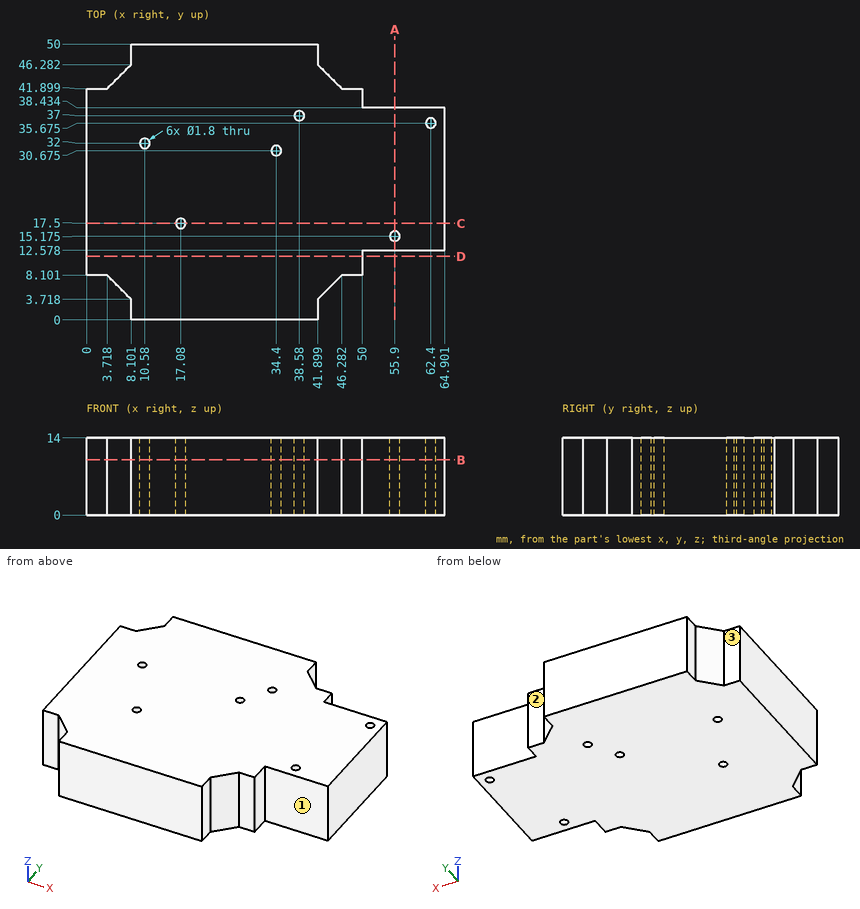
Job drawing, mm, ordinate dimensions from the low corner. One solid piece. A direction names the side the tool comes from. Give positions to 0.01 mm unless a question says otherwise; leave off trailing zeros. Loops run counter-clockwise (first coordinate to the right, second up) from the corner with the lowest first, then second, coordinate; pieces in that order, holes last. Notation, with made-up numbers: M 61.5,64 L 119.5,64 A18 ccw 119.5,96 Z; hole C 19.25,45.25 d1. An arc over 180 degrees is marked long. Put each result on its own line as item: value. Start each with the question number.
1) Saw through at D-D (y = 11.5). List the corners of the cut face in (x, z).
2) Saw through at A-A (x = 55.9). List the corners of the cut face in (y, z) (1 decimal).
3) Saw through at C-C (y = 17.5). List the corners of the cut face in (x, z).
4) 3-axis set-ups, long thin cutter, end or side, ignore diameter. For the marked faces 1, 2 and 3: which of +Z, -Z, +X, -X, +Y, -Y reach the whole face in a straight line?
5) Flat gauge pins, fed straight in: pin 1 (1.6 mm diameter, centred on x = 17.08, y = 17.5, fed in from +Z); pin 2 (4 mm diameter, centred on x = 47.5, z = 9, fed in from +Y); pin 3 (4 mm diameter, centred on y = 48.5, z = 7.5, fed in from -X); pin 4 (1.1 mm diameter, centred on x = 2, z = 9, fed in from -Y). Where does each tip first touch, or does it go through?
6) Probe probe 1 along Y at (x, z) = (17.08, 6); probe 2 along Y at (x, z) = (62.4, 6.75) (1 decimal); probe 3 along X at (y, z) = (30.5, 5.25). List the from-to ranges inside material, lowest first.
7) Saw through at B-B (z = 10). List the corners of the cut face in (x, y) (1 decimal).
Numbers:
1. outline: M 0,0 L 50,0 L 50,14 L 0,14 Z
2. outline: M 12.6,0 L 14.3,0 L 14.3,14 L 12.6,14 Z; M 16.1,0 L 38.4,0 L 38.4,14 L 16.1,14 Z
3. outline: M 0,0 L 16.18,0 L 16.18,14 L 0,14 Z; M 17.98,0 L 64.9,0 L 64.9,14 L 17.98,14 Z
4. face 1: +Z, -Z, +X, -Y
4. face 2: +Z, -Z, +X, +Y
4. face 3: +Z, -Z, -X, +Y
5. pin 1: through
5. pin 2: y = 42.68
5. pin 3: x = 8.1
5. pin 4: y = 8.1
6. probe 1: 0 to 16.6, 18.4 to 50
6. probe 2: 12.6 to 34.8, 36.6 to 38.4
6. probe 3: 0 to 33.52, 35.28 to 64.9
7. outline: M 0,8.1 L 3.7,8.1 L 8.1,3.7 L 8.1,0 L 41.9,0 L 41.9,3.7 L 46.3,8.1 L 50,8.1 L 50,12.6 L 64.9,12.6 L 64.9,38.4 L 50,38.4 L 50,41.9 L 46.3,41.9 L 41.9,46.3 L 41.9,50 L 8.1,50 L 8.1,46.3 L 3.7,41.9 L 0,41.9 Z; hole C 10.6,32 d1.8; hole C 17.1,17.5 d1.8; hole C 34.4,30.7 d1.8; hole C 38.6,37 d1.8; hole C 55.9,15.2 d1.8; hole C 62.4,35.7 d1.8
